Design review of the part built by this model. Coordinates are the model's own, in mm. A direction names the side the tool comes from. Round coordinates to 2 decimals unless told otherwise and drop trailing zeros. Loops run counter-clockwise (first coordinate to the right, second up) from the corner with the lowest first, then second, coordinate; pieces in that order, holes last. Notation, with made-up numbers: (-33, 58.25) - (-21, 58.25) arc R15 ccw to (-21, 84.25) - close; hole circle Ø8 at (63.25, 28.25). An arc over 180 degrees is marked (long way). Answer as CSV lines item,"result". Start each with the question number.
(1) Wall thickness on L1, parallel to X at y = -15, z = -9.25; L2, parallel to Z at x = 4, y = 2.25; L3, parallel to Y at x = -1, z = -9: over which ranges is each line inside the solid? List them lowest first.
(2) Consider section C-C (x = -6.5). Give the boundary of the cut face in (y, z) (3 decimals).
(3) For P1, Ø5.5, axis at x = -2, z = -3.5, coming from the +Y side; P2, Ø2.5, axis at x = -6.5, y = -15.12, coming from the +Z side, all flat-tipped, find the tip position at first contact; note any pin that passes through.
(4) Consider section B-B (z = -6). Give the boundary of the cut face in (x, y).
(5) For faces 1 (the flat face through (-1, -5, -12)), 2 (the flat face through (-1, 8.5, -6)), list the 3-axis set-ups (+Z, -Z, +X, -X, +Y, -Y) from which the entire face can be reached by the end or side of a thin tool; tool diameter is ignored.
(6) Mouldability with a two-part tool opening along X and no side actions: class faces 3 (the cylindrical face through (-7.6, -14.1, -5.9)), 4 (the flat face through (8, -5, -6)), 5 (the flat face through (-1, 9, -11.375)) as released by +X, released by -X, zero draft, split by the parting line, or undercut.
(7) Consider section D-D (z = -3.25). Give the boundary of the cut face in (x, y), and give its area (3 significant figures).
(8) Consider section A-A (y = -15.12). Give the boundary of the cut face in (x, z).
from build123d import *

# Parameters (mm, degrees)
BOSS_EXTRUDE1_DEPTH = 8
CUT_EXTRUDE1_REACH  = 12
SKETCH3_R           = 1
BOSS_EXTRUDE2_DEPTH = 10
SKETCH7_W           = 18
SKETCH7_H           = 12
SKETCH7_R           = 1
BOSS_EXTRUDE3_DEPTH = 21.12
SKETCH11_R          = 1.5
CUT_EXTRUDE4_DEPTH  = 13


with BuildPart() as part:
    # Sketch2 → Boss-Extrude1 (new body)
    with BuildSketch(Plane(origin=(0, 0, 0), x_dir=(0, 0, -1), z_dir=(1, 0, 0))):
        Polygon((0, 0), (0, 10), (0.625, 10), (0.625, 8.5), (11.375, 8.5), (11.375, 10), (12, 10), (12, 0), align=None)
    extrude(amount=BOSS_EXTRUDE1_DEPTH)

    # Sketch3 → Cut-Extrude1 (cut, up to next)
    with BuildSketch(Plane.XZ, mode=Mode.PRIVATE) as cut_extrude1_sk1:
        with Locations((4, -6)):
            Circle(SKETCH3_R)
    cut_extrude1_tool1 = extrude(cut_extrude1_sk1.sketch, amount=-CUT_EXTRUDE1_REACH, mode=Mode.PRIVATE) & part.part
    add(cut_extrude1_tool1.solids().sort_by_distance((4, 0, -6))[0], mode=Mode.SUBTRACT)

    # Sketch6 → Boss-Extrude2 (add)
    with BuildSketch(Plane.ZY):
        Polygon((-12, 0), (0, 0), (0, 10), (-0.625, 10), (-0.625, 8.5), (-11.375, 8.5), (-11.375, 10), (-12, 10), align=None)
    extrude(amount=BOSS_EXTRUDE2_DEPTH)

    # Sketch7 → Boss-Extrude3 (add)
    with BuildSketch(Plane.XZ):
        with Locations((-1, -6)):
            Rectangle(SKETCH7_W, SKETCH7_H)
        with Locations((4, -6)):
            Circle(SKETCH7_R, mode=Mode.SUBTRACT)
    extrude(amount=BOSS_EXTRUDE3_DEPTH)

    # Sketch11 → Cut-Extrude4 (cut, through all)
    with BuildSketch(Plane.XY):
        with Locations((-6.5, -15.12)):
            Circle(SKETCH11_R)
        with Locations((-1, -17.12)):
            Circle(SKETCH11_R)
    extrude(amount=-CUT_EXTRUDE4_DEPTH, mode=Mode.SUBTRACT)


solid = part.part
Determined:
1,L1,"x = -10 to -8, -5 to 8"
1,L2,"z = -12 to -7, -5 to 0"
1,L3,"y = -21.12 to -18.62, -15.62 to 8.5"
2,outline,"(-21.12, -12) - (-16.62, -12) - (-16.62, 0) - (-21.12, 0) - close; (-13.62, -12) - (10, -12) - (10, -11.375) - (8.5, -11.375) - (8.5, -0.625) - (10, -0.625) - (10, 0) - (-13.62, 0) - close"
3,P1,"stops at y = 8.5"
3,P2,"passes through"
4,outline,"(-10, -21.12) - (3, -21.12) - (3, 8.5) - (-10, 8.5) - close; (5, -21.12) - (8, -21.12) - (8, 8.5) - (5, 8.5) - close; hole circle Ø3 at (-6.5, -15.12); hole circle Ø3 at (-1, -17.12)"
5,face 1,"-Z, +X, -X, +Y, -Y"
5,face 2,"+X, -X, +Y"
6,face 3,"undercut"
6,face 4,"released by +X"
6,face 5,"zero draft"
7,outline,"(-10, -21.12) - (8, -21.12) - (8, 8.5) - (-10, 8.5) - close; hole circle Ø3 at (-6.5, -15.12); hole circle Ø3 at (-1, -17.12)"
7,area,"519 mm^2"
8,outline,"(-10, -12) - (-8, -12) - (-8, 0) - (-10, 0) - close; (-5, -12) - (8, -12) - (8, 0) - (-5, 0) - close; hole circle Ø2 at (4, -6)"
